Model file for the job. Use its own axes, mm. A direction names the side the tool comes from. Round coordinates to 2 decimals unless told otherwise and drop trailing zeros. Loops run counter-clockwise (first coordinate to the right, second up) from the corner with the lowest first, then second, coordinate; pieces in that order, holes last. Notation, with made-up numbers: M 45.5,-13.5 L 101.5,-13.5 A21 cw 101.5,14.5 Z; hole C 77.5,50.5 d11. An arc over 180 degrees is marked long. Answer in a Markdown table with one row per item.
Autodesk Inventor part; units mm, degrees
ref_plane "YZ Plane" through (0, 0, 0) normal (1, 0, 0) x (0, 1, 0)
ref_plane "XZ Plane" through (0, 0, 0) normal (0, 1, 0) x (-1, 0, 0)
ref_plane "XY Plane" through (0, 0, 0) normal (0, 0, 1) x (1, 0, 0)
sketch "Sketch1" plane through (0, 0, 0) normal (0, 0, 1) x (1, 0, 0)
  line L0 (-15.05, -11.5) -> (15.05, -11.5)
  line L1 (15.05, -11.5) -> (15.05, 11.5)
  line L2 (15.05, 11.5) -> (-15.05, 11.5)
  line L3 (-15.05, 11.5) -> (-15.05, -11.5)
  line L4 (-15.05, -11.5) -> (15.05, 11.5) construction
  line L5 (15.05, -11.5) -> (-15.05, 11.5) construction
  point P0 (0, 0)
  dimension "d0" = 30.1
  dimension "d1" = 23
extrude "Plate1" add sketch "Sketch1" along normal blind 1.5
sketch "Sketch6" plane through (0, 0, 1.5) normal (0, 0, 1) x (1, 0, 0)
  circle A0 centre (-8.15, 8.43) radius 0.7835
  circle A1 centre (-8.15, -7.57) radius 0.7835
  circle A2 centre (5.07, 7.43) radius 0.7835
  circle A3 centre (5.07, -6.57) radius 0.7835
  circle A4 centre (12.37, 0.43) radius 0.7835
  point P0 (0, 0)
hole "Hole2" at (-8.15, 8.43, 1.5) at (5.07, 7.43, 1.5) at (12.37, 0.43, 1.5) at (5.07, -6.57, 1.5) at (-8.15, -7.57, 1.5) direction (0, 0, -1) diameter 2.1 end through all
sketch "Sketch7" plane through (0, 0, 1.5) normal (0, 0, 1) x (1, 0, 0)
  circle A0 centre (-15.05, 0.43) radius 6.4
  circle A1 centre (-15.05, 0.43) radius 6.55
  point P0 (0, 0)
  dimension "d42" = 0.15
extrude "Cut1" cut sketch "Sketch7" against normal blind 1.5 contours A0 | A1
sketch "Sketch8" plane through (15.05, -10, 0) normal (0, -1, 0) x (1, 0, 0)
  line L0 (-30.1, 0) -> (0, 0)
  line L1 (0, 0) -> (0, 20)
  line L2 (0, 20) -> (-30.1, 20)
  line L3 (-30.1, 20) -> (-30.1, 0)
edge flange "Flange2" height 20 angle 90 thickness 1.5 bend radius 0.31 thickness toward (0, -1, 0) relief tear relief width 1.5 relief depth 0.75 edges at (0, -11.5, 1.5) wall of the first edge with corners at (-15.05, -10, 0) (15.05, -10, 0) (15.05, -10, 20) (-15.05, -10, 20)
bend "Bend2"
corner "Corner2"
sketch "Sketch9" plane through (-15.05, -10, 20) normal (0, 1, 0) x (1, 0, 0)
  circle A0 centre (10.05, 40.25) radius 40
  circle A1 centre (10.05, 40.25) radius 50
  point P0 (15.05, 20)
  dimension "d39" = 10
extrude "Cut2" cut sketch "Sketch9" against normal blind 1.5
fillet "Corner Round1" radius 1 2 edges at (15.05, 11.5, 0.75) (-15.05, 11.5, 0.75)
sketch "Sketch10" plane through (-15.05, -10, 1.81) normal (0, 1, 0) x (1, 0, 0)
  line L0 (30.1, 0) -> (0, 0)
  arc A0 (0, -16.6569) -> (30.1, -12.5521) centre (10.05, 22.06) ccw
  line L1 (15.05, 0) -> (15.05, -17.6263) construction
  point P0 (15.05, 1.81)
  point P1 (6.05, -5)
  point P2 (24.05, -5)
  point P3 (24.05, -12.5)
  point P4 (6.05, -14.5)
  dimension "d44" = 18
  dimension "d45" = 9.5
  dimension "d46" = 7.5
  dimension "d47" = 5
hole "Hole3" at (-9, -10, 6.81) at (9, -10, 6.81) at (9, -10, 14.31) at (-9, -10, 16.31) direction (0, -1, 0) diameter 2.1 end through all
equation "\"d27\" = Thickness"
equation "\"d40\" = Thickness"
equation "\"d2\" = Thickness"
equation "\"d29\" = BendReliefWidth"
equation "\"d30\" = BendReliefDepth"
equation "\"d31\" = MinimumRemnant"
equation "\"d32\" = TransitionRadius"
equation "\"d35\" = BendRadius"
equation "\"d36\" = CornerReliefSize"
equation "\"d37\" = GapSize"
equation "\"d38\" = JacobiRadiusSize"
equation "\"BendReliefWidth\" = Thickness"
equation "\"BendReliefDepth\" = 0.5 * Thickness"
equation "\"CornerReliefSize\" = 4 * Thickness"
equation "\"MinimumRemnant\" = 2 * Thickness"
equation "\"TransitionRadius\" = BendRadius"
equation "\"JacobiRadiusSize\" = BendRadius"
equation "\"GapSize\" = Thickness"
properties part number "axis_2_bottom_L_frame(top)" material "Aluminum 6061-AHC"
1. Pin check, flat tips, straight feed: pin 1 (2.5 mm diameter, centred on x = 9, z = 6.81, fed in from +Y); pin 2 (8 mm diameter, centred on x = 8.5, y = -5.5, fed in from +Z). Stop position of each tip, or through.
Verdict:
| item | result |
|---|---|
| pin 1 | stops at y = -10 |
| pin 2 | stops at z = 1.5 |
2. Wall check: probe 1 along Y at (x, z) = (-8.15, 0.7); probe 2 along Y at (x, z) = (5.07, 0.55); probe 3 along Y at (x, z) = (-3, 5.5). Give the ranges that are in metal, low to high.
Verdict:
| item | result |
|---|---|
| probe 1 | y = -11.12 to -8.62, -6.52 to 7.38, 9.48 to 11.5 |
| probe 2 | y = -10.99 to -7.62, -5.52 to 6.38, 8.48 to 11.5 |
| probe 3 | y = -11.5 to -10 |
3. Saw through at B-B (z = 16.5). Write the cut outline in (x, y), and give its area (3 significant figures).
Verdict:
| item | result |
|---|---|
| outline | M -15.05,-11.5 L -10.03,-11.5 L -10.03,-10 L -15.05,-10 Z; M -7.97,-11.5 L 10.79,-11.5 L 10.79,-10 L -7.97,-10 Z |
| area | 35.7 mm² |
4. Saw through at A-A (y = 1). Write the cut outline in (x, z), and give its area (3 significant figures).
Verdict:
| item | result |
|---|---|
| outline | M -8.52,0 L 11.49,0 L 11.49,1.5 L -8.52,1.5 Z; M 13.25,0 L 15.05,0 L 15.05,1.5 L 13.25,1.5 Z |
| area | 32.7 mm² |
5. Saw through at C-C (x = -4). Write the cut outline in (y, z), and give its area (3 significant figures).
Verdict:
| item | result |
|---|---|
| outline | M -11.5,1.81 A1.81 ccw -9.69,0 L 11.5,0 L 11.5,1.5 L -9.69,1.5 A0.31 cw -10,1.81 L -10,19.74 L -11.5,19.74 Z |
| area | 61.2 mm² |
6. Mould opens along Y. For faces 1 (the cylindrical face through (4.75, -7.57, 0.74)), 2 (the cylindrical face through (14.765, 11.199, 0.76)), 3 (the cylindrical face through (8.11, -10.76, 14.87)), 4 (the cylindrical face through (-8.5, 0.3, 0.8)) say: +Y half, -Y half, draft (parallel to the pull), parting line (faces both ways), or undercut.
Verdict:
| item | result |
|---|---|
| face 1 | undercut |
| face 2 | +Y half |
| face 3 | draft |
| face 4 | undercut |
7. Saw through at D-D (z = 8.75). Write the cut outline in (x, y), and give its area (4 significant figures).
Verdict:
| item | result |
|---|---|
| outline | M -15.05,-11.5 L 15.05,-11.5 L 15.05,-10 L -15.05,-10 Z |
| area | 45.15 mm² |
8. Tool access for faces 5 (the flat face through (0, 1, 0)), 6 (the flat face through (0, -10, 11)): list every direction of +Z, -Z, +X, -X, +Y, -Y with a clear straight run to the whole face (end or side of a thin tool).
Verdict:
| item | result |
|---|---|
| face 5 | -Z, +X, -X, +Y, -Y |
| face 6 | +Z, +X, -X, +Y |
